from build123d import *

# Parameters (mm, degrees)
ESQUISSE2_R             = 10
BOSS_EXTRU_2_DEPTH      = 40
ESQUISSE3_R             = 7.25
ENL_V_MAT_EXTRU_1_DEPTH = 30
CONG_2_R                = 2


with BuildPart() as part:
    # Esquisse2 → Boss.-Extru.2 (new body)
    with BuildSketch(Plane(origin=(0, 0, 0), x_dir=(1, 0, 0), z_dir=(0, 1, 0))):
        Circle(ESQUISSE2_R)
    extrude(amount=BOSS_EXTRU_2_DEPTH)

    # Esquisse3 → Enlèv. mat.-Extru.1 (cut)
    with BuildSketch(Plane.XZ):
        Circle(ESQUISSE3_R)
    extrude(amount=-ENL_V_MAT_EXTRU_1_DEPTH, mode=Mode.SUBTRACT)

    # Congé2
    cong_2_edges = [part.edges().sort_by_distance(p)[0] for p in [
        (-7.25, 30, 0),
    ]]
    fillet(cong_2_edges, radius=CONG_2_R)

    # Esquisse9 → Révolution7 (revolve)
    with BuildSketch(Plane(origin=(0, 0, 0), x_dir=(0, 0, -1), z_dir=(1, 0, 0))):
        with BuildLine():
            Line((20, 57.326780647), (-20, 57.326780647))
            ThreePointArc((-20, 57.326780647), (0, 37.326780647), (20, 57.326780647))
        make_face()
    revolve(axis=Axis((0, 57.326780647, -20), (0, 0, 1)))


solid = part.part
Check sheet for the modelled part. Datum: model origin and axes. Units: mm. Coordinates: 2 decimals unless noted, no trailing zeros. Loops run counter-clockwise (first coordinate to the right, second up) from the corner with the lowest first, then second, coordinate; pieces in that order, holes last. Notation, with made-up numbers: (82.5, -34.5) -> (106.5, -34.5) arc R24 cw to (106.5, 0.5) -> close; hole circle Ø4 at (-17.75, 72). An arc over 180 degrees is marked (long way). Write item = value, one per line. Start each with the question number.
1. Depth check by flat-ended pin: P1, Ø3, axis at x = 1.5, z = -2.5, coming from the -Y side; P2, Ø1, axis at x = -6, y = 38.5, coming from the +Z side; P3, Ø4, axis at y = 17.5, z = 3, coming from the -X side. Enter the tip coordinate at first touch or a pass-through.
2. Draft check along Z on faces 1 (the cylindrical face through (3.35, 13.8, -6.43)), 2 (the flat face through (7, 0, -3)), 3 (the cylindrical face through (-2.17, 19.72, 9.76)). Enter one of: released by +Z, released by -Z, zero draft, split by the parting line, or undercut.
3. Section check D-D on z = 12.5. Record the cut outline in (x, y).
4. Material ranges on line 1 (Z direction, x = 0, y = 9); line 2 (X direction, y = 25.5, z = 4); line 3 (Z direction, x = 8.5, y = 17.5), recorded low to high.
5. Section check C-C on y = 41.5. Record the cut outline in (x, z), then the cut area to 3 significant figures.
Responses:
q1.P1 = 30
q1.P2 = 8.35
q1.P3 = -9.95
q2.face_1 = undercut
q2.face_2 = zero draft
q2.face_3 = split by the parting line
q3.outline = circle Ø31.22 at (0, 57.33)
q4.line_1 = -10 to -7.25, 7.25 to 10
q4.line_2 = -9.17 to -6.05, 6.05 to 9.17
q4.line_3 = -5.27 to 5.27
q5.outline = circle Ø24.46 at (0, 0)
q5.area = 470 mm2
